Verification items for this drawing (mm, ordinates from the low corner). A direction names the side the tool comes from. Coordinates: 2 decimals unless noted, no trailing zeros. Loops run counter-clockwise (first coordinate to the right, second up) from the corner with the lowest first, then second, coordinate; pieces in that order, holes last. Notation, with made-up numbers: M 28.25,87.25 L 69.25,87.25 A17 cw 69.25,107.25 Z; hole C 68,16.25 d5. An arc over 180 degrees is marked long. Use CSV: the item, a comma, the result in double quotes.
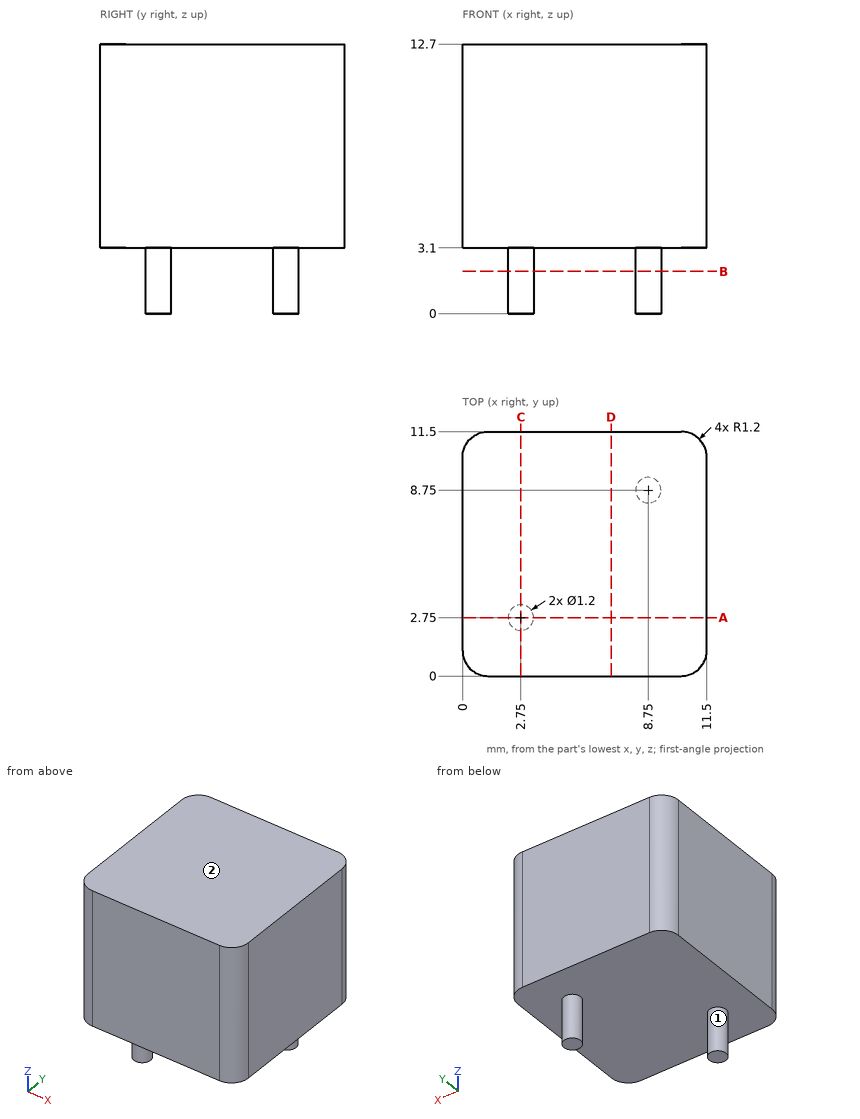
1. Section check A-A, the plane y = 2.75. Record the cut outline in (x, z).
The answers:
outline,"M 0,3.1 L 2.15,3.1 L 2.15,0 L 3.35,0 L 3.35,3.1 L 11.5,3.1 L 11.5,12.7 L 0,12.7 Z"
2. Gauge pin test, flat end, axial feed: P1, Ø3.5, axis at x = 3, y = 7, coming from the -Z side. Record the tip position at first contact, or that the pin passes through.
The answers:
P1,"z = 3.1"
3. Section check B-B, the plane z = 2. Record the cut outline in (x, y), plus the area to 3 significant figures.
The answers:
outline,"C 2.75,2.75 d1.2; C 8.75,8.75 d1.2"
area,"2.26 mm^2"
4. Thickness scan on line 1 (Z direction, x = 3.5, y = 6); line 2 (Y direction, x = 10.75, z = 5.75); line 3 (Y direction, x = 8.5, z = 2). Record the ranges inside material, lowest first. Write a range as [from, to].
The answers:
line 1,"[3.1, 12.7]"
line 2,"[0.09, 11.41]"
line 3,"[8.2, 9.3]"
5. Set-up check for the marked faces 1 and 2: record each of +Z, -Z, +X, -X, +Y, -Y from which the full face is reachable in a straight line by a thin tool's end or side.
The answers:
face 1,"-Z"
face 2,"+Z, +X, -X, +Y, -Y"
6. Section check D-D, the plane x = 7. Record the cut outline in (y, z).
The answers:
outline,"M 0,3.1 L 11.5,3.1 L 11.5,12.7 L 0,12.7 Z"
